```python
from build123d import *

# Parameters (mm, degrees)
SKETCH_1_R      = 9
SKETCH_1_R_2    = 7.5
EXTRUDE_2_DEPTH = 400
SKETCH_3_R      = 10
SKETCH_3_R_2    = 8.5
EXTRUDE_3_DEPTH = 18
FILLET_2_R      = 1


with BuildPart() as part:
    # 草圖1 → 填料-伸長2 (new body)
    with BuildSketch(Plane(origin=(0, 0, 0), x_dir=(0, 0, -1), z_dir=(1, 0, 0))):
        Circle(SKETCH_1_R)
        Circle(SKETCH_1_R_2, mode=Mode.SUBTRACT)
    extrude(amount=EXTRUDE_2_DEPTH)

    # 草圖3 → 填料-伸長3 (add)
    with BuildSketch(Plane.ZY.offset(18)):
        Circle(SKETCH_3_R)
        Circle(SKETCH_3_R_2, mode=Mode.SUBTRACT)
    extrude(amount=-EXTRUDE_3_DEPTH)

    # 圓角2
    fillet_2_edges = [part.edges().sort_by_distance(p)[0] for p in [
        (0, 0, -10),
    ]]
    fillet(fillet_2_edges, radius=FILLET_2_R - 0.0001)  # a hair under: the kernel refuses the full size


solid = part.part
```
The model under review builds one solid part; all positions refer to its coordinate system, in mm. A direction names the side the tool comes from. Round coordinates to 2 decimals unless told otherwise and drop trailing zeros. Loops run counter-clockwise (first coordinate to the right, second up) from the corner with the lowest first, then second, coordinate; pieces in that order, holes last. Notation, with made-up numbers: (60, 25) - (112, 25) arc R25 cw to (112, 63) - close; hole circle Ø2 at (-38.75, 84.25). An arc over 180 degrees is marked (long way). Write each question's results on one line, items separated by ' | '. Start each with the question number.
Q1. Insertion check: P1, Ø3, axis at x = 352.5, z = -5.5, coming from the -Y side; P2, Ø2, axis at x = 118.5, y = -7, coming from the +Z side; P3, Ø5, axis at x = 30, y = 7, coming from the +Z side. Each pin has a flat end and moves straight along its axis. Give the tip position at first contact, or say it passes through.
Q2. Wall thickness on line 1 along Y through (x, z) = (-7.75, 0); line 2 along Y through (x, z) = (148, 0); line 3 along Z through (x, y) = (93.5, -0.75): over which ranges is each line inside the solid? List them lowest first. Write a range as [from, to].
Q3. Tool access review of faces 4 (the cylindrical face through (-9.126, 7.167, 4.57)), 5 (the cylindrical face through (-9.62, -9.76, -2.17)): name each direction out of +Z, -Z, +X, -X, +Y, -Y from which nothing blocks a thin tool from reaching the whole face with its end or side.
Q4. Draft analysis for pull direction Y (two halves, no side actions). For faces 1 (the flat face through (0, -8, 0)), 2 (the cylindrical face through (197.2, 8.923, 1.172)), 3 (the flat face through (-18, -7.4, -4.5)), state which applies: pulls with the +Y half, pulls with the -Y half, needs draft (parallel to the pull), parting line crosses it, or undercut.
Q5. Take a section at C-C on x = 29.5. Give the boundary of the cut face in (y, z).
Data:
1) P1: stops at y = -8.06 | P2: stops at z = 6.71 | P3: stops at z = 7.79
2) line 1: y = [-10, -8.5], [8.5, 10] | line 2: y = [-9, -7.5], [7.5, 9] | line 3: z = [-8.97, -7.46], [7.46, 8.97]
3) face 4: -X | face 5: +X, -X
4) face 1: undercut | face 2: parting line crosses it | face 3: needs draft
5) outline: circle Ø18 at (0, 0); hole circle Ø15 at (0, 0)
